The drawing under review shows one solid part. Ordinate dimensions are in mm from its lowest x, y, z. Coordinates: 2 decimals unless noted, no trailing zeros. Write each loop counter-clockwise with the first axis right and the second up, starting at its lowest first coordinate (ties: lowest second). Pieces come first, ordered by that corner, then holes. Notation, with made-up numbers: (-3, 55.5) - (29, 55.5) arc R25 ccw to (29, 68.5) - close; hole circle Ø6 at (58.25, -25). An arc over 180 degrees is marked (long way). Put each result on its own line as item: value. Start each with the question number.
Item 1: Consider section D-D on y = 209.5. Give the boundary of the cut face in (x, z).
Item 2: Consider section C-C on z = 7.5. Give the boundary of the cut face in (x, y).
Item 3: For pin 1 (12 mm diameter, centred on y = 152, z = 24, fed in from -X); pin 2 (12 mm diameter, centred on y = 145.5, z = 24, fed in from +X), all flat-tipped, find the tip position at first contact; note any pin that passes through.
Item 4: Mouldability with a two-part tool opening along X and no side actions: class the marked faces 1, 2 and 3 as pulls with the +X half, pulls with the -X half, needs draft (parallel to the pull), parting line crosses it, or undercut.
Item 5: Consider section B-B on x = 279.5. Give the boundary of the cut face in (y, z), then the cut area to 3 significant figures.
Item 6: To check wall thickness, follow L1, parallel to X at y = 196.5, z = 24; L2, parallel to Y at x = 283, z = 27; L3, parallel to Z at x = 385, y = 34.5. State the ranges of each line that lie inside material, in increasing order. Write a range as [from, to].
Item 7: Consider section A-A on y = 178. Give the boundary of the cut face in (x, z), then the cut area to 3 significant figures.
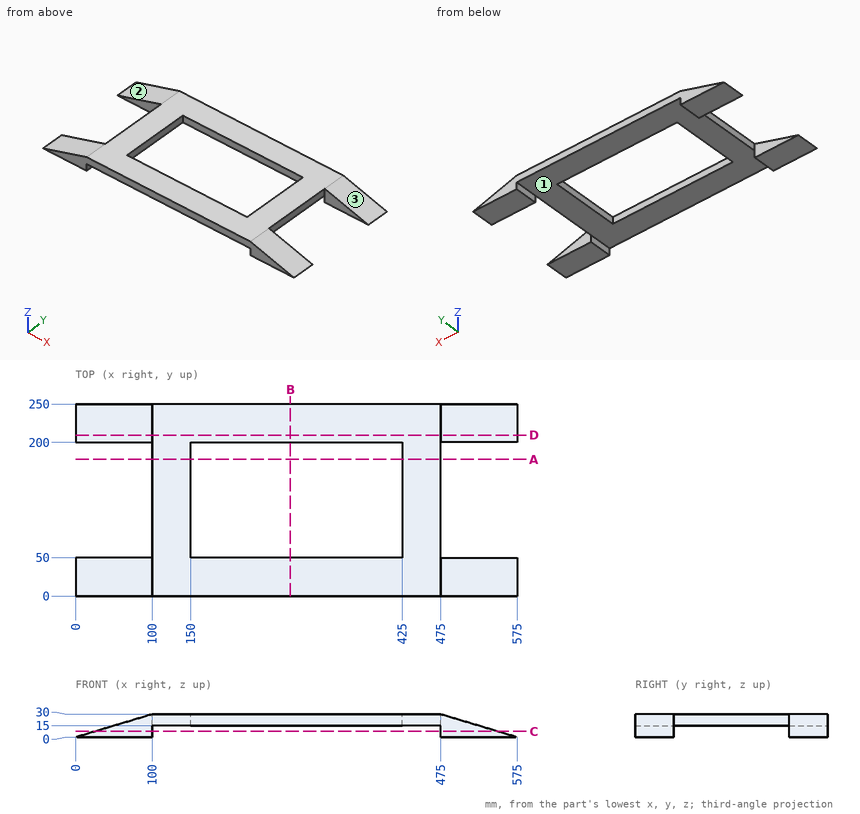
Report:
1. outline: (0, 0) - (100, 0) - (100, 15) - (475, 15) - (475, 0) - (575, 0) - (475, 30) - (100, 30) - close
2. outline: (25, 0) - (100, 0) - (100, 50) - (25, 50) - close; (25, 200) - (100, 200) - (100, 250) - (25, 250) - close; (475, 0) - (550, 0) - (550, 50) - (475, 50) - close; (475, 200) - (550, 200) - (550, 250) - (475, 250) - close
3. pin 1: x = 100
3. pin 2: x = 475
4. face 1: undercut
4. face 2: pulls with the -X half
4. face 3: pulls with the +X half
5. outline: (0, 15) - (50, 15) - (50, 30) - (0, 30) - close; (200, 15) - (250, 15) - (250, 30) - (200, 30) - close
5. area: 1,500 mm²
6. L1: [100, 150], [425, 475]
6. L2: [0, 50], [200, 250]
6. L3: [15, 30]
7. outline: (100, 15) - (150, 15) - (150, 30) - (100, 30) - close; (425, 15) - (475, 15) - (475, 30) - (425, 30) - close
7. area: 1,500 mm²
